from build123d import *

# Parameters (mm, degrees)
F0_W     = 914.4
F0_H     = 914.4
F1_DEPTH = 25.4
F2_R     = 7.62
F3_DEPTH = 457.2
F5_DEPTH = 914.4


with BuildPart() as f1:
    # F0 (on Right) → F1 (new body)
    with BuildSketch(Plane.YZ):
        Rectangle(F0_W, F0_H)
    extrude(amount=F1_DEPTH)

    # F2 (on Front) → F3 (join, through all)
    with BuildSketch(Plane.XZ):
        with BuildLine():
            Line((0, -435.864), (-14.732, -435.864))
            ThreePointArc((-14.732, -435.864), (-25.4, -446.532), (-14.732, -457.2))
            Line((-14.732, -457.2), (0, -457.2))
            Line((0, -457.2), (0, -435.864))
        make_face()
        with Locations((-14.732, -446.532)):
            Circle(F2_R, mode=Mode.SUBTRACT)
    extrude(amount=F3_DEPTH)

    # F4 (on face) → F5 (cut, through all)
    with BuildSketch(Plane.XZ.offset(457.2)):
        with BuildLine():
            ThreePointArc((25.4, -425.6636202335), (15.2344848329, -443.4731324002), (0, -457.2))
            Line((0, -457.2), (25.4, -457.2))
            Line((25.4, -457.2), (25.4, -425.6636202335))
        make_face()
    extrude(amount=-F5_DEPTH, mode=Mode.SUBTRACT)


solid = f1.part
The listing builds one solid part. Answer for the finished solid, in the listing's coordinates (mm). A direction names the side the tool comes from. Give positions to 0.01 mm unless a question says otherwise; leave off trailing zeros. Order: outer loops, then holes, each group sorted by start corner. A loop starts at its lowest first (then second) coordinate and runs counter-clockwise, first axis right, second up. Notation, with made-up numbers: (80.25, 85) - (113.25, 85) arc R17 cw to (113.25, 89) - close; hole circle Ø8 at (-32.5, -15.75). An arc over 180 degrees is marked (long way). One line per item, written item: value. Start each with the question number.
1) Given pin 1 Ø5 at (y, z) = (144.5, -204.5) entering from -X; pin 2 Ø9 at (x, z) = (-14.732, -446.532) entering from +Y; pin 3 Ø6.5 at (x, z) = (-11, -451) entering from +Y; pin 4 Ø4.5 at (x, y) = (-4.5, -162) entering from +Z, each flat-ended and moving along its own axis, determine where each tip first touches the part or whether it passes through.
2) A cutting plane is placed at A-A on y = -184. Give the vertices of the cut face in (x, z), then the cut area to 3 significant figures.
3) Find the intervals of material crossed by L1, parallel to Z at x = -13, y = -172; L2, parallel to Z at x = -21.5, y = -239.5; L3, parallel to X at y = -93, z = -60.5, in increasing order.
4) A tool of negligible diameter and unlimited length cuts with its end or side. For faces 1 (the face through (13, 457.2, -6)), 2 (the face through (-7, 0, -449)), from which of +Z, -Z, +X, -X, +Y, -Y can it reach the whole face along a straight path? Write none if from no direction.
5) A cutting plane is placed at C-C on y = 263. Give the vertices of the cut face in (x, z), then the cut area to 3 significant figures.
6) A cutting plane is placed at B-B on z = 126.5. Give the vertices of the cut face in (x, y).
Answer sheet:
1. pin 1: stops at x = 0
1. pin 2: passes through
1. pin 3: stops at y = 0
1. pin 4: stops at z = -435.86
2. outline: (-14.73, -457.2) - (0, -457.2) arc R64.61 ccw to (25.4, -425.66) - (25.4, 457.2) - (0, 457.2) - (0, -435.86) - (-14.73, -435.86) arc R10.67 ccw to start; hole circle Ø15.24 at (-14.73, -446.53)
2. area: 23,200 mm2
3. L1: z = -457.2 to -453.95, -439.11 to -435.86
3. L2: z = -454.78 to -450.03, -443.03 to -438.29
3. L3: x = 0 to 25.4
4. face 1: +Z, -Z, +X, -X, +Y
4. face 2: +Z, -Z, -X, +Y
5. outline: (0, -457.2) arc R64.61 ccw to (25.4, -425.66) - (25.4, 457.2) - (0, 457.2) - close
5. area: 22,900 mm2
6. outline: (0, -457.2) - (25.4, -457.2) - (25.4, 457.2) - (0, 457.2) - close
